CAD build for the part. Positions are in the model's coordinates, mm. Face numbers are marked on the shaded views. A direction names the side the tool comes from. Coordinates: 2 decimals unless noted, no trailing zeros. Write item = value, one per line. Start each with the question number.
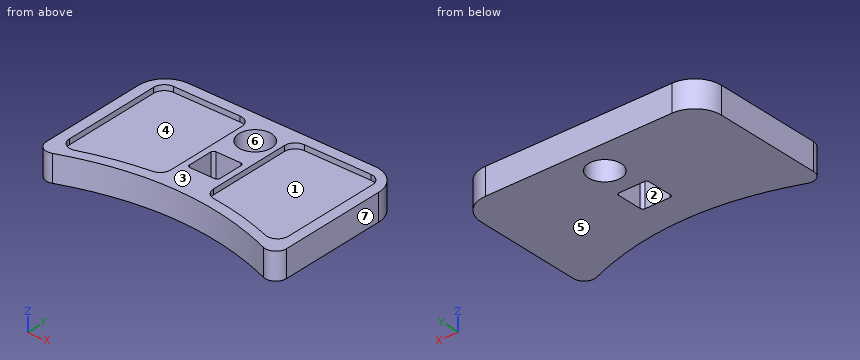
```python
from build123d import *

# Parameters (mm, degrees)
BOSS_EXTRUDE1_DEPTH = 5
SKETCH2_R           = 3.05
SKETCH2_W           = 5.7
SKETCH2_H           = 5.7
CUT_EXTRUDE1_DEPTH  = 29.419018875
FILLET1_R           = 0.5
CUT_EXTRUDE2_DEPTH  = 1
FILLET2_R           = 5
FILLET3_R           = 2
FILLET4_R           = 2


with BuildPart() as part:
    # Sketch1 → Boss-Extrude1 (new body)
    with BuildSketch(Plane.XY):
        with BuildLine():
            Line((-22.5, -11.625), (-22.5, -16.625))
            add(Edge.make_bspline(
                [(-22.5, -16.625), (0, -6.625), (22.5, -16.625)],
                knots=[0, 0, 0, 1, 1, 1], degree=2))
            Line((22.5, -16.625), (22.5, -11.625))
            Line((22.5, -11.625), (22.5, 11.625))
            Line((22.5, 11.625), (-22.5, 11.625))
            Line((-22.5, 11.625), (-22.5, -11.625))
        make_face()
    extrude(amount=-BOSS_EXTRUDE1_DEPTH)

    # Sketch2 → Cut-Extrude1 (cut, through all)
    with BuildSketch(Plane.XY):
        with Locations((0, 5.875)):
            Circle(SKETCH2_R)
        with Locations((0, -2.875)):
            Rectangle(SKETCH2_W, SKETCH2_H)
    extrude(amount=-CUT_EXTRUDE1_DEPTH, mode=Mode.SUBTRACT)

    # Fillet1
    fillet1_edges = [part.edges().sort_by_distance(p)[0] for p in [
        (2.85, -0.025, -2.5),
        (2.85, -5.725, -2.5),
        (-2.85, -5.725, -2.5),
        (-2.85, -0.025, -2.5),
    ]]
    fillet(fillet1_edges, radius=FILLET1_R)

    # Sketch3 → Cut-Extrude2 (cut)
    with BuildSketch(Plane.XY):
        with BuildLine():
            Line((-20.5, 9.625), (-20.5, -13.775617284))
            add(Edge.make_bspline(
                [(-4, -9.783024691), (-9.5, -10.217592593), (-15, -11.54845679), (-20.5, -13.775617284)],
                knots=[0.588888889, 0.588888889, 0.588888889, 0.588888889, 0.955555556, 0.955555556, 0.955555556, 0.955555556], degree=3))
            Line((-4, -9.783024691), (-4, 9.625))
            Line((-4, 9.625), (-20.5, 9.625))
        make_face()
        with BuildLine():
            Line((4, 9.625), (4, -9.783024691))
            add(Edge.make_bspline(
                [(4, -9.783024691), (9.5, -10.217592593), (15, -11.54845679), (20.5, -13.775617284)],
                knots=[0.588888889, 0.588888889, 0.588888889, 0.588888889, 0.955555556, 0.955555556, 0.955555556, 0.955555556], degree=3))
            Line((20.5, -13.775617284), (20.5, 9.625))
            Line((20.5, 9.625), (4, 9.625))
        make_face()
    extrude(amount=-CUT_EXTRUDE2_DEPTH, mode=Mode.SUBTRACT)

    # Fillet2
    fillet2_edges = [part.edges().sort_by_distance(p)[0] for p in [
        (-22.5, 11.625, -2.5),
        (22.5, 11.625, -2.5),
    ]]
    fillet(fillet2_edges, radius=FILLET2_R)

    # Fillet3
    fillet3_edges = [part.edges().sort_by_distance(p)[0] for p in [
        (22.5, -16.625, -2.5),
        (-22.5, -16.625, -2.5),
    ]]
    fillet(fillet3_edges, radius=FILLET3_R)

    # Fillet4
    fillet4_edges = [part.edges().sort_by_distance(p)[0] for p in [
        (20.5, -13.775617284, -0.5),
        (4, -9.783024691, -0.5),
        (20.5, 9.625, -0.5),
        (4, 9.625, -0.5),
        (-4, 9.625, -0.5),
        (-20.5, 9.625, -0.5),
        (-4, -9.783024691, -0.5),
        (-20.5, -13.775617284, -0.5),
    ]]
    fillet(fillet4_edges, radius=FILLET4_R)


solid = part.part
```
1. Probe L1, parallel to Y at x = 0, z = -2.75 (3 decimals); L2, parallel to X at y = 9.25, z = -0.6; L3, parallel to Z at x = 6, y = -8. List the from-to ranges inside material, lowest first.
2. 3-axis set-ups, long thin cutter, end or side, ignore diameter. For the marked faces 1, 2 and 3: which of +Z, -Z, +X, -X, +Y, -Y reach the whole face in a straight line?
3. Flat gauge pins, fed straight in: pin 1 (0.8 mm diameter, centred on x = 14, z = -0.5, fed in from -Y); pin 2 (1.1 mm diameter, centred on x = -14.5, z = -0.5, fed in from -Y); pin 3 (6 mm diameter, centred on x = -0.5, y = 8, fed in from +Z); pin 4 (8 mm diameter, centred on x = 14.5, y = 4.5, fed in from +Z). Where does each tip first touch, or does it go through?
4. Mould opens along X. For the marked faces 4, 5, 6 and 7 say: released by +X, released by -X, zero draft, split by the parting line, or undercut.
5. Slice it at A-A (x = 0). Give the number of separate pieces and of enclosed holes in the cut face, plus the area to 4 significant figures.
Calculated:
q1.L1 = -11.625 to -5.725, -0.025 to 2.825, 8.925 to 11.625
q1.L2 = -21.76 to -19.67, -4.83 to 4.83, 19.67 to 21.76
q1.L3 = -5 to -1
q2.face_1 = +Z
q2.face_2 = +Z, -Z
q2.face_3 = +Z, +X, -X, +Y, -Y
q3.pin_1 = -13.67
q3.pin_2 = -13.86
q3.pin_3 = 0
q3.pin_4 = -1
q4.face_4 = undercut
q4.face_5 = zero draft
q4.face_6 = undercut
q4.face_7 = released by +X
q5.separate_pieces = 3
q5.enclosed_holes = 0
q5.area = 57.25 mm²
